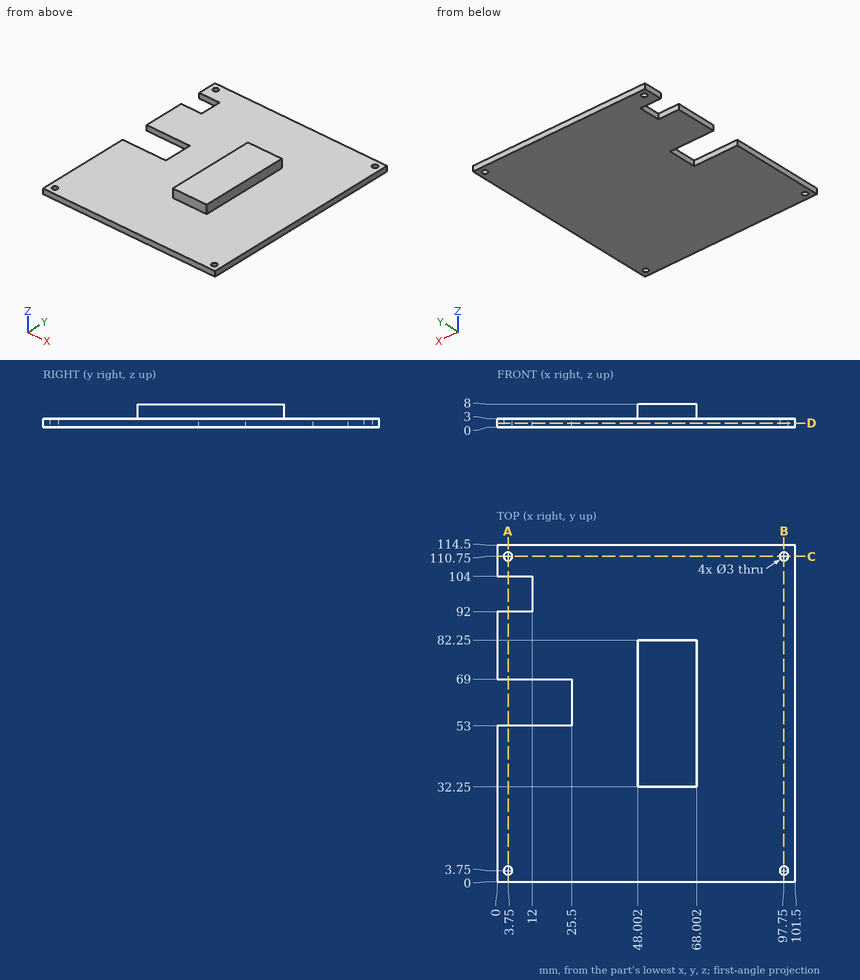
Drawing for the job (mm, zero at the part's lowest x, y, z). Round coordinates to 2 decimals unless told otherwise and drop trailing zeros. Loops run counter-clockwise (first coordinate to the right, second up) from the corner with the lowest first, then second, coordinate; pieces in that order, holes last. Notation, with made-up numbers: (-32.5, 5) -> (-5.5, 5) arc R18 ccw to (-5.5, 14) -> close; hole circle Ø3 at (53, 2.25). An arc over 180 degrees is marked (long way). Answer as CSV lines item,"result". Start each with the question number.
1) Slice it at D-D (z = 1.5). List the corners of the cut face in (x, y), plus the area to 3 significant figures.
2) Probe line 1 along Y through (x, z) = (3.75, 2.4); line 2 along Y through (x, z) = (97.75, 2.15); line 3 along X through (y, z) = (110.75, 0.75). List the from-to ranges inside material, lowest first.
3) Slice it at A-A (x = 3.75). List the corners of the cut face in (y, z).
4) Slice it at C-C (y = 110.75). List the corners of the cut face in (x, z).
5) Slice it at B-B (x = 97.75). List the corners of the cut face in (y, z).
6) Pin check, flat tips, straight feed: P1, Ø3.5, axis at y = 62, z = 1, coming from the -X side; P2, Ø1.5, axis at y = 96.5, z = 1, coming from the -X side; P3, Ø1.5, axis at y = 65, z = 5.5, coming from the -X side; P4, Ø1.8, axis at x = 3.75, y = 110.75, coming from the +Z side. Stop position of each tip, or through.
Filled in:
1,outline,"(0, 0) -> (101.5, 0) -> (101.5, 114.5) -> (0, 114.5) -> (0, 104) -> (12, 104) -> (12, 92) -> (0, 92) -> (0, 69) -> (25.5, 69) -> (25.5, 53) -> (0, 53) -> close; hole circle Ø3 at (3.75, 3.75); hole circle Ø3 at (3.75, 110.75); hole circle Ø3 at (97.75, 3.75); hole circle Ø3 at (97.75, 110.75)"
1,area,"11,000 mm2"
2,line 1,"y = 0 to 2.25, 5.25 to 53, 69 to 92, 104 to 109.25, 112.25 to 114.5"
2,line 2,"y = 0 to 2.25, 5.25 to 109.25, 112.25 to 114.5"
2,line 3,"x = 0 to 2.25, 5.25 to 96.25, 99.25 to 101.5"
3,outline,"(0, 0) -> (2.25, 0) -> (2.25, 3) -> (0, 3) -> close; (5.25, 0) -> (53, 0) -> (53, 3) -> (5.25, 3) -> close; (69, 0) -> (92, 0) -> (92, 3) -> (69, 3) -> close; (104, 0) -> (109.25, 0) -> (109.25, 3) -> (104, 3) -> close; (112.25, 0) -> (114.5, 0) -> (114.5, 3) -> (112.25, 3) -> close"
4,outline,"(0, 0) -> (2.25, 0) -> (2.25, 3) -> (0, 3) -> close; (5.25, 0) -> (96.25, 0) -> (96.25, 3) -> (5.25, 3) -> close; (99.25, 0) -> (101.5, 0) -> (101.5, 3) -> (99.25, 3) -> close"
5,outline,"(0, 0) -> (2.25, 0) -> (2.25, 3) -> (0, 3) -> close; (5.25, 0) -> (109.25, 0) -> (109.25, 3) -> (5.25, 3) -> close; (112.25, 0) -> (114.5, 0) -> (114.5, 3) -> (112.25, 3) -> close"
6,P1,"stops at x = 25.5"
6,P2,"stops at x = 12"
6,P3,"stops at x = 48"
6,P4,"passes through"
